from build123d import *

# Parameters (mm, degrees)
SKETCH1_R           = 3
BOSS_EXTRUDE1_DEPTH = 3
SKETCH2_R           = 3
CUT_EXTRUDE1_DEPTH  = 3
SKETCH3_W           = 9
SKETCH3_H           = 9
BOSS_EXTRUDE2_DEPTH = 3
BOSS_EXTRUDE3_DEPTH = 12


with BuildPart() as part:
    # Sketch1 → Boss-Extrude1 (new body)
    with BuildSketch(Plane(origin=(0, 0, 0), x_dir=(1, 0, 0), z_dir=(0, 1, 0))):
        with BuildLine():
            Line((-3.269734365, -7.845727727), (-3.269734365, 9.654272273))
            ThreePointArc((-3.269734365, 9.654272273), (1.730265635, 14.654272273), (6.730265635, 9.654272273))
            Line((6.730265635, 9.654272273), (6.730265635, -7.845727727))
            ThreePointArc((6.730265635, -7.845727727), (1.730265635, -12.845727727), (-3.269734365, -7.845727727))
        make_face()
        with Locations((1.730265635, -7.845727727)):
            Circle(SKETCH1_R, mode=Mode.SUBTRACT)
    extrude(amount=BOSS_EXTRUDE1_DEPTH)

    # Sketch2 → Cut-Extrude1 (cut)
    with BuildSketch(Plane(origin=(0, 3, 0), x_dir=(1, 0, 0), z_dir=(0, 1, 0))):
        with Locations((1.730265635, 9.654272273)):
            Circle(SKETCH2_R)
    extrude(amount=-CUT_EXTRUDE1_DEPTH, mode=Mode.SUBTRACT)

    # Sketch3 → Boss-Extrude2 (add)
    with BuildSketch(Plane(origin=(0, 0, 0), x_dir=(-1, 0, 0), z_dir=(0, -1, 0))):
        with BuildLine():
            Line((-1.730265635, 14.654272273), (16.269734365, 14.654272273))
            Line((16.269734365, 14.654272273), (16.269734365, 1.654272273))
            Line((16.269734365, 1.654272273), (3.269734365, 1.654272273))
            Line((3.269734365, 1.654272273), (3.269734365, 9.654272273))
            ThreePointArc((3.269734365, 9.654272273), (1.805268271, 13.189806179), (-1.730265635, 14.654272273))
        make_face()
        with Locations((9.769734365, 8.154272273)):
            Rectangle(SKETCH3_W, SKETCH3_H, mode=Mode.SUBTRACT)
    extrude(amount=-BOSS_EXTRUDE2_DEPTH)

    # Sketch4 → Boss-Extrude3 (add)
    with BuildSketch(Plane(origin=(0, 0, 0), x_dir=(-1, 0, 0), z_dir=(0, -1, 0))):
        Polygon((5.269734365, 12.654272273), (5.269734365, 14.654272273), (16.269734365, 14.654272273), (16.269734365, 1.654272273), (5.269734365, 1.654272273), (5.269734365, 3.654272273), (14.269734365, 3.654272273), (14.269734365, 12.654272273), align=None)
    extrude(amount=BOSS_EXTRUDE3_DEPTH)


solid = part.part
Verification items for the finished model (mm, model axes). A direction names the side the tool comes from. Give positions to 0.01 mm unless a question says otherwise; leave off trailing zeros. Order: outer loops, then holes, each group sorted by start corner. A loop starts at its lowest first (then second) coordinate and runs counter-clockwise, first axis right, second up. Notation, with made-up numbers: M 46,-31.5 L 78,-31.5 A17 ccw 78,-8.5 Z; hole C -29,11.25 d5. An arc over 180 degrees is marked long. Use one line per item in the form item = value. Start each with the question number.
Q1. Mould release check, pull along Z, two halves, no side actions. Record for faces 1 (the flat face through (-9, -3, -14.654)), 2 (the flat face through (-5.27, 1, -8)), 3 (the flat face through (-16.27, -4, -8)): +Z half, -Z half, draft (parallel to the pull), parting line (faces both ways), or undercut.
Q2. Section check C-C (x = 4). Enter the section's corners in (y, z).
Q3. Section check D-D (z = 10.5). Enter the section's corners in (x, y).
Q4. Go/stop test with flat-tipped pins: pin 1 Ø1 at (y, z) = (-3.5, -2) entering from +X; pin 2 Ø6 at (x, z) = (-2, 8.5) entering from -Y; pin 3 Ø8 at (x, y) = (-13, -4.5) entering from +Z; pin 4 Ø6 at (x, z) = (-6.5, 2.5) entering from +Y. Record where each tip stops, or that it passes through.
Q5. Scan lines: line 1 along Z through (x, y) = (-9.25, 1.75); line 2 along X through (y, z) = (-2.25, -12); line 3 along Y through (x, z) = (4, 2.25). Record each from-to range of solid material in increasing order. Write a range as [from, to].
Q6. Section check B-B (y = 1.5). Enter the section's corners in (x, z).
Q7. Access from +Z, -Z, +X, -X, +Y, -Y to the whole of each face (thin tool, end or side, straight path). Record for faces 4 (the flat face through (1, 0, -1)), 5 (the flat face through (-3.27, 1, 3)), 6 (the flat face through (-10, -4, -12.654)), 7 (the flat face through (-2, 3, -4)).
Q8. Section check A-A (x = -9.5). Enter the section's corners in (y, z), then the cut area to 3 significant figures.
Evaluation:
q1.face_1 = -Z half
q1.face_2 = undercut
q1.face_3 = draft
q2.outline = M 0,-14.11 L 3,-14.11 L 3,-11.62 L 0,-11.62 Z; M 0,-7.69 L 3,-7.69 L 3,5.88 L 0,5.88 Z; M 0,9.81 L 3,9.81 L 3,12.3 L 0,12.3 Z
q3.outline = M -2.51,0 L 0.33,0 L 0.33,3 L -2.51,3 Z; M 3.13,0 L 5.97,0 L 5.97,3 L 3.13,3 Z
q4.pin_1 = -5.27
q4.pin_2 = 0
q4.pin_3 = -1.65
q4.pin_4 = through
q5.line_1 = [-14.65, -12.65], [-3.65, -1.65]
q5.line_2 = [-16.27, -14.27]
q5.line_3 = [0, 3]
q6.outline = M -16.27,-14.65 L 1.73,-14.65 A5 ccw 6.73,-9.65 L 6.73,7.85 A5 ccw -3.27,7.85 L -3.27,-1.65 L -16.27,-1.65 Z; hole M -14.27,-12.65 L -5.27,-12.65 L -5.27,-3.65 L -14.27,-3.65 Z; hole C 1.73,-9.65 d6; hole C 1.73,7.85 d6
q7.face_4 = +Z, -Z, +X, -Y
q7.face_5 = +Z, -X, +Y, -Y
q7.face_6 = +Y, -Y
q7.face_7 = +Z, -Z, +X, -X, +Y
q8.outline = M -12,-14.65 L 3,-14.65 L 3,-12.65 L -12,-12.65 Z; M -12,-3.65 L 3,-3.65 L 3,-1.65 L -12,-1.65 Z
q8.area = 60.0 mm2
